```python
from build123d import *

# Parameters (mm, degrees)
F2_R     = 3.02334
F3_DEPTH = 59.549888


with BuildPart() as f1:
    # F0 (on Front) → F1 (revolve)
    with BuildSketch(Plane.XZ):
        Polygon((-59.548888, 10.583334), (0, 10.583334), (0, 26.105555), (-3.386669, 26.105555), (-3.386669, 40.216666), (-13.828888, 40.216666), (-13.828888, 23.00111), (-59.548888, 23.00111), align=None)
    revolve(axis=Axis((-68.222322, 0, 0), (-1, 0, 0)))

    # F2 (on face) → F3 (cut, through all)
    with BuildSketch(Plane.YZ):
        with Locations((0, 10.583334)):
            Circle(F2_R)
    extrude(amount=-F3_DEPTH, mode=Mode.SUBTRACT)


solid = f1.part
```
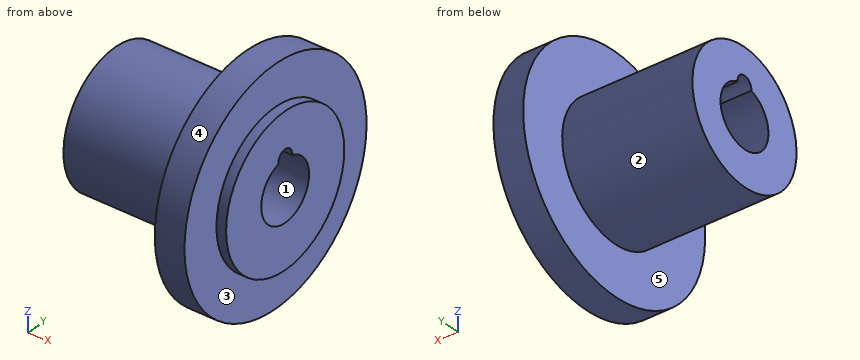
The listing builds one solid part. Answer for the finished solid, in the listing's coordinates (mm). Face numbers are marked on the shaded views. A direction names the side the tool comes from. Coordinates: 2 decimals unless noted, no trailing zeros. Loops run counter-clockwise (first coordinate to the right, second up) from the corner with the lowest first, then second, coordinate; pieces in that order, holes last. Notation, with made-up numbers: M 27,-31 L 86,-31 A26 ccw 86,-13 Z; hole C 72,62.5 d2. An arc over 180 degrees is marked long. Answer as a JSON object with one key per item and string values. Group by question number.
Item 1: Section D-D (z = -16.5) is taken. Write down the section's boundary in (x, y).
Item 2: Section A-A (z = 0) is taken. Write down the section's boundary in (x, y), and give its area (3 significant figures).
Item 3: Section C-C (x = -27) is taken. Write down the section's boundary in (y, z), and give its area (3 significant figures).
Item 4: Each of these flat-tipped pins is pushed along its axis until it touches: P1, Ø3, axis at x = -23.5, y = -5.5, coming from the +Z side; P2, Ø4, axis at y = 7, z = -4.5, coming from the -X side; P3, Ø2, axis at x = -45.5, z = -20, coming from the +Y side; P4, Ø2, axis at x = -37, z = -2, coming from the +Y side. Where does it stop, or does it pass through?
Item 5: Section B-B (y = 0) is taken. Write down the section's boundary in (x, z).
Item 6: Consider L1, parallel to X at y = -35.5, z = 1.5; L2, parallel to Y at x = -54, z = -3.5; L3, parallel to Z at x = -54, y = 7.5. Determine where each line is inside the solid, lowest interval first.
Item 7: Determine the mould class of the marked faces 1, 2 and 3 for opening direction Y: +Y half, -Y half, draft (parallel to the pull), parting line (faces both ways), or undercut.
Item 8: Which of the six approach directions +Z, -Z, +X, -X, +Y, -Y give full straight-line access (tool end or side, diameter ignored) to the marked faces 4 and 5?
Solved:
{
 "1": {"outline": "M -59.55,-16.03 L -13.83,-16.03 L -13.83,-36.68 L -3.39,-36.68 L -3.39,-20.23 L 0,-20.23 L 0,20.23 L -3.39,20.23 L -3.39,36.68 L -13.83,36.68 L -13.83,16.03 L -59.55,16.03 Z"},
 "2": {"outline": "M -59.55,-23 L -13.83,-23 L -13.83,-40.22 L -3.39,-40.22 L -3.39,-26.11 L 0,-26.11 L 0,-10.58 L -59.55,-10.58 Z; M -59.55,10.58 L 0,10.58 L 0,26.11 L -3.39,26.11 L -3.39,40.22 L -13.83,40.22 L -13.83,23 L -59.55,23 Z", "area": "1,860 mm2"},
 "3": {"outline": "C 0,0 d46; hole M -2.99,10.15 A10.58 ccw long 2.99,10.15 A3.02 ccw long Z", "area": "1,290 mm2"},
 "4": {"P1": "stops at z = 22.65", "P2": "passes through", "P3": "stops at y = 12.96", "P4": "stops at y = 22.98"},
 "5": {"outline": "M -59.55,-23 L -13.83,-23 L -13.83,-40.22 L -3.39,-40.22 L -3.39,-26.11 L 0,-26.11 L 0,-10.58 L -59.55,-10.58 Z; M -59.55,13.61 L 0,13.61 L 0,26.11 L -3.39,26.11 L -3.39,40.22 L -13.83,40.22 L -13.83,23 L -59.55,23 Z"},
 "6": {"L1": "x = -13.83 to -3.39", "L2": "y = -22.73 to -9.99, 9.99 to 22.73", "L3": "z = -21.74 to -7.47, 7.47 to 21.74"},
 "7": {"face 1": "undercut", "face 2": "parting line", "face 3": "draft"},
 "8": {"face 4": "+X, -X", "face 5": "-X"}
}
